Part model, mm, in its own coordinate system. A direction names the side the tool comes from. Give positions to 0.01 mm unless a question says otherwise; leave off trailing zeros. Write each loop counter-clockwise with the first axis right and the second up, starting at its lowest first coordinate (ties: lowest second). Pieces come first, ordered by that corner, then holes. Notation, with made-up numbers: M 31.5,46 L 49.5,46 A19 ccw 49.5,70 Z; hole C 27,53.25 d1. An arc over 180 degrees is marked long. Use CSV: the item, a comma, the result in double quotes. Start each with the question number.
1. Band-saw the part on D-D, the plane x = -20. List the corners of the cut face in (y, z), then the cut area to 3 significant figures.
2. 3-axis set-ups, long thin cutter, end or side, ignore diameter. For faces 1 (the face through (8, 5, 39)), 2 (the face through (-1.172, 8.923, 19.227)): which of +Z, -Z, +X, -X, +Y, -Y reach the whole face in a straight line?
3. Band-saw the part on B-B, the plane y = 0. List the corners of the cut face in (x, z).
4. Band-saw the part on A-A, the plane x = 0. List the corners of the cut face in (y, z).
5. Drop flat-ended pins along their axis: pin 1 Ø4 at (x, z) = (1.5, 19.5) entering from +Y; pin 2 Ø5 at (x, z) = (-2.5, 13) entering from -Y; pin 3 Ø4 at (x, z) = (-15.5, 26.5) entering from +Y. Give the stop position or say it passes through.
6. Mould opens along Y. For faces 3 (the face through (-29.97, 1.32, 22.18)), 4 (the face through (-20.21, -9.15, 22.18)), 5 (the face through (6, 7, 0)) say: pulls with the +Y half, pulls with the -Y half, needs draft (parallel to the pull), parting line crosses it, or undercut.
7. Band-saw the part on C-C, the plane z = 14. List the corners of the cut face in (x, y) (3 decimals).
8. Drill centre lines: line 1 along Y through (x, z) = (0, 12); line 2 along Y through (x, z) = (0, 43); line 3 along Y through (x, z) = (-21, 31.5). Where is each one in solid material? Low to high. Write a range as from..to.
from build123d import *

# Parameters (mm, degrees)
SKETCH1_R            = 30
SKETCH1_R_2          = 9
BOSS_EXTRUDE1_DEPTH  = 45
M5_CLEARANCE_HOLE1_D = 5.5
SKETCH4_R            = 10.5
CUT_EXTRUDE1_DEPTH   = 6


with BuildPart() as part:
    # Sketch1 → Boss-Extrude1 (new body)
    with BuildSketch(Plane.XY):
        Circle(SKETCH1_R)
        Circle(SKETCH1_R_2, mode=Mode.SUBTRACT)
    extrude(amount=BOSS_EXTRUDE1_DEPTH)

    # M5 Clearance Hole1 (through all)
    with Locations(Plane.XY.offset(45)):
        with Locations((0, 23.75), (20.56810334, 11.875), (20.56810334, -11.875), (0, -23.75), (-20.56810334, -11.875), (-20.56810334, 11.875), (0, 0)):
            Hole(M5_CLEARANCE_HOLE1_D / 2)

    # Sketch4 → Cut-Extrude1 (cut)
    with BuildSketch(Plane.XY.offset(45)):
        Circle(SKETCH4_R)
    extrude(amount=-CUT_EXTRUDE1_DEPTH, mode=Mode.SUBTRACT)


solid = part.part
Output:
1,outline,"M -22.36,0 L -14.57,0 L -14.57,45 L -22.36,45 Z; M -9.18,0 L 9.18,0 L 9.18,45 L -9.18,45 Z; M 14.57,0 L 22.36,0 L 22.36,45 L 14.57,45 Z"
1,area,"1,530 mm²"
2,face 1,"+Z"
2,face 2,"+Z, -Z"
3,outline,"M -30,0 L -9,0 L -9,39 L -10.5,39 L -10.5,45 L -30,45 Z; M 9,0 L 30,0 L 30,45 L 10.5,45 L 10.5,39 L 9,39 Z"
4,outline,"M -30,0 L -26.5,0 L -26.5,45 L -30,45 Z; M -21,0 L -9,0 L -9,39 L -10.5,39 L -10.5,45 L -21,45 Z; M 9,0 L 21,0 L 21,45 L 10.5,45 L 10.5,39 L 9,39 Z; M 26.5,0 L 30,0 L 30,45 L 26.5,45 Z"
5,pin 1,"stops at y = 30"
5,pin 2,"stops at y = -30"
5,pin 3,"stops at y = 26.79"
6,face 3,"parting line crosses it"
6,face 4,"undercut"
6,face 5,"needs draft"
7,outline,"C 0,0 d60; hole C -20.568,-11.875 d5.5; hole C -20.568,11.875 d5.5; hole C 0,0 d18; hole C 0,-23.75 d5.5; hole C 0,23.75 d5.5; hole C 20.568,-11.875 d5.5; hole C 20.568,11.875 d5.5"
8,line 1,"y = -30..-26.5, -21..-9, 9..21, 26.5..30"
8,line 2,"y = -30..-26.5, -21..-10.5, 10.5..21, 26.5..30"
8,line 3,"y = -21.42..-14.59, -9.16..9.16, 14.59..21.42"
